Design review of the part shown in the three views and the two pictorial views. Dimensions are in mm from the part's minimum x, y and z. A direction names the side the tool comes from. Give positions to 0.01 mm unless a question says otherwise; leave off trailing zeros. Order: outer loops, then holes, each group sorted by start corner. A loop starts at its lowest first (then second) coordinate and runs counter-clockwise, first axis right, second up. Notation, with made-up numbers: (-8, 13.5) - (-3, 13.5) arc R11 ccw to (-3, 27.5) - close; hole circle Ø5 at (74, -38.5). An arc over 180 degrees is marked (long way). Put each result on its own line as item: value.
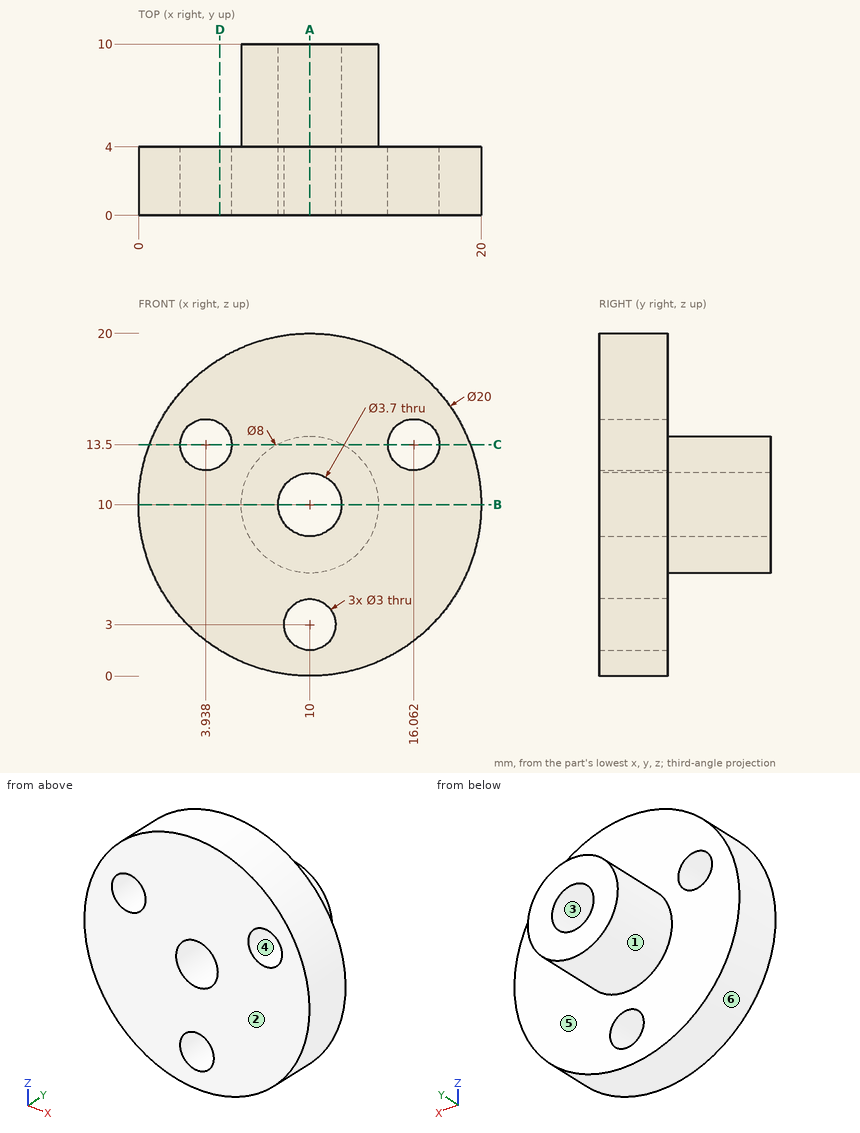
(1) The part is to be moulded in two halves that separate along X. For the marked faces 3, 4, 5 and 6, say which applies: pulls with the +X half, pulls with the -X half, needs draft (parallel to the pull), parting line crosses it, or undercut.
The answers:
face 3: undercut
face 4: undercut
face 5: needs draft
face 6: parting line crosses it
(2) Clearance check with flat-ended pins moving along their axes: pin 1 Ø5 at (y, z) = (3, 18) entering from -X; pin 2 Ø6 at (x, y) = (11.5, 8.5) entering from +Z; pin 3 Ø5 at (y, z) = (7.5, 5.5) entering from -X. State where each tip first meets the part, or that it passes through.
The answers:
pin 1: x = 1.65
pin 2: z = 14
pin 3: x = 6.54
(3) Take a section at D-D, the plane x = 4.75. Write out the cut boundary in (y, z).
The answers:
outline: (0, 1.49) - (4, 1.49) - (4, 12.24) - (0, 12.24) - close; (0, 14.76) - (4, 14.76) - (4, 18.51) - (0, 18.51) - close
(4) Take a section at B-B, the plane z = 10. Write out the cut boundary in (x, y), then the cut area to 3 significant figures.
The answers:
outline: (0, 0) - (8.15, 0) - (8.15, 10) - (6, 10) - (6, 4) - (0, 4) - close; (11.85, 0) - (20, 0) - (20, 4) - (14, 4) - (14, 10) - (11.85, 10) - close
area: 91.0 mm^2
(5) Wall thickness on L1, parallel to Y at x = 16.75, z = 11.75; L2, parallel to X at y = 8, z = 10; L3, parallel to Z at x = 10.75, y = 3.75: over which ranges is each line inside the solid? List them lowest first.
The answers:
L1: 0 to 4
L2: 6 to 8.15, 11.85 to 14
L3: 0.03 to 1.7, 4.3 to 8.31, 11.69 to 19.97
(6) Take a section at A-A, the plane x = 10. Write out the cut boundary in (y, z).
The answers:
outline: (0, 0) - (4, 0) - (4, 1.5) - (0, 1.5) - close; (0, 4.5) - (4, 4.5) - (4, 6) - (10, 6) - (10, 8.15) - (0, 8.15) - close; (0, 11.85) - (10, 11.85) - (10, 14) - (4, 14) - (4, 20) - (0, 20) - close
(7) Take a section at C-C, the plane z = 13.5. Write out the cut boundary in (x, y).
The answers:
outline: (0.63, 0) - (2.44, 0) - (2.44, 4) - (0.63, 4) - close; (5.44, 0) - (14.56, 0) - (14.56, 4) - (11.94, 4) - (11.94, 10) - (8.06, 10) - (8.06, 4) - (5.44, 4) - close; (17.56, 0) - (19.37, 0) - (19.37, 4) - (17.56, 4) - close
(8) For the marked faces 1 and 2, list the 3-axis set-ups (+Z, -Z, +X, -X, +Y, -Y) from which the entire face can be reached by the end or side of a thin tool; tool diameter is ignored.
The answers:
face 1: +Y
face 2: +Z, -Z, +X, -X, -Y
